Part model, mm, in its own coordinate system. A direction names the side the tool comes from. Coordinates: 2 decimals unless noted, no trailing zeros. Write each loop counter-clockwise with the first axis right and the second up, starting at its lowest first coordinate (ties: lowest second). Pieces come first, ordered by that corner, then holes. Notation, with made-up numbers: M -3.75,-35 L 41.25,-35 A32 ccw 41.25,-2 Z; hole C -40,-30 d9. An arc over 180 degrees is marked long. Use a Markdown table: item, result. Add a question column.
Q1. Tool access for faces 1 (the flat face through (-131, -28.775, -2)), 2 (the flat face through (2, -56.825, -2)), 3 (the flat face through (9.525, 52, -2)): list every direction of +Z, -Z, +X, -X, +Y, -Y with a clear straight run to the whole face (end or side of a thin tool).
Q2. Mould opens along X. For faces 4 (the flat face through (-143.075, 10, -2)), 5 (the cylindrical face through (-150, -54.8, -2.5)), 6 (the cylindrical face through (150.1, -54.7, -2.5)) say: released by +X, released by -X, zero draft, split by the parting line, or undercut.
Q3. Slice it at B-B on x = 129. Write the cut outline in (y, z) (3 decimals).
Q4. Pin check, flat tip, straight feed: pin 1 Ø4.5 at (x, y) = (147.575, -19.05) entering from +Z. Stop position of the tip, or through.
Q5. Slice it at C-C on z = -3.6. Count the separate pieces of the cut face and the enclosed holes in it, then the cut area to 3 significant figures.
Q6. Wall check: L1, parallel to Y at x = 19.05, z = -2.8 (3 decimals); L2, parallel to X at y = -19, z = -1.6 (3 decimals); L3, parallel to Y at x = 88, z = -4.35 (3 decimals). Give the ranges that are in metal, low to high. Write a range as from..to.
Q7. Slice it at A-A on y = 32. Write the cut outline in (x, z) (3 decimals), then the cut area to 3 significant figures.
from build123d import *

# Parameters (mm, degrees)
PAD001_DEPTH  = 5
FILLET004_R   = 7
FILLET005_R   = 1
FILLET006_R   = 1.2
SKETCH014_R   = 1.7
HOLE003_DEPTH = 25


with BuildPart() as part:
    # Sketch001 → Pad001 (new body)
    with BuildSketch(Plane.XY):
        Polygon((-9.525, 56.825), (-9.525, 47.825), (-143.075, 47.825), (-143.075, -28.775), (-119.2625, -28.775), (-119.2625, -47.825), (100.2125, -47.825), (100.2125, -28.775), (143.075, -28.775), (143.075, 47.825), (9.525, 47.825), (9.525, 56.825), (152.075, 56.825), (152.075, -56.825), (-152.075, -56.825), (-152.075, 56.825), align=None)
    extrude(amount=-PAD001_DEPTH)

    # Fillet004
    fillet004_edges = [part.edges().sort_by_distance(p)[0] for p in [
        (-152.075, 56.825, -2.5),
        (-152.075, -56.825, -2.5),
        (152.075, 56.825, -2.5),
        (152.075, -56.825, -2.5),
    ]]
    fillet(fillet004_edges, radius=FILLET004_R)

    # Fillet005
    fillet005_edges = [part.edges().sort_by_distance(p)[0] for p in [
        (-143.075, 47.825, -2.5),
        (-143.075, -28.775, -2.5),
        (-119.2625, -47.825, -2.5),
        (100.2125, -47.825, -2.5),
        (143.075, -28.775, -2.5),
        (143.075, 47.825, -2.5),
    ]]
    fillet(fillet005_edges, radius=FILLET005_R)

    # Fillet006
    fillet006_edges = [part.edges().sort_by_distance(p)[0] for p in [
        (100.2125, -28.775, -2.5),
        (-119.2625, -28.775, -2.5),
    ]]
    fillet(fillet006_edges, radius=FILLET006_R)

    # Sketch014 (on Face1 of Fillet006) → Hole003 (cut)
    with BuildSketch(Plane.XY):
        with Locations((147.575, 52.325)):
            Circle(SKETCH014_R)
        with Locations((147.575, -19.05)):
            Circle(SKETCH014_R)
        with Locations((95.25, -52.325)):
            Circle(SKETCH014_R)
        with Locations((-95.25, -52.325)):
            Circle(SKETCH014_R)
        with Locations((-147.575, -19.05)):
            Circle(SKETCH014_R)
        with Locations((-147.575, 52.325)):
            Circle(SKETCH014_R)
        with Locations((-19.05, 52.325)):
            Circle(SKETCH014_R)
        with Locations((19.05, 52.325)):
            Circle(SKETCH014_R)
    extrude(amount=-HOLE003_DEPTH, mode=Mode.SUBTRACT)


solid = part.part
Recorded:
| question | item | result |
|---|---|---|
| 1 | face 1 | +Z, -Z |
| 1 | face 2 | +Z, -Z, +X, -X, -Y |
| 1 | face 3 | +Z, -Z, +Y |
| 2 | face 4 | undercut |
| 2 | face 5 | released by -X |
| 2 | face 6 | released by +X |
| 3 | outline | M -56.825,-5 L -28.775,-5 L -28.775,0 L -56.825,0 Z; M 47.825,-5 L 56.825,-5 L 56.825,0 L 47.825,0 Z |
| 4 | pin 1 | z = 0 |
| 5 | separate pieces | 1 |
| 5 | enclosed holes | 8 |
| 5 | area | 8,180 mm² |
| 6 | L1 | -56.825..-47.825, 47.825..50.625, 54.025..56.825 |
| 6 | L2 | -152.075..-149.274, -145.876..-143.075, 143.075..145.876, 149.274..152.075 |
| 6 | L3 | -56.825..-47.825, 47.825..56.825 |
| 7 | outline | M -152.075,-5 L -143.075,-5 L -143.075,0 L -152.075,0 Z; M 143.075,-5 L 152.075,-5 L 152.075,0 L 143.075,0 Z |
| 7 | area | 90.0 mm² |
